Build history of the part. All positions in model axes, mm. A direction names the side the tool comes from. Give positions to 0.01 mm unless a question says otherwise; leave off trailing zeros. Write each loop counter-clockwise with the first axis right and the second up, starting at its lowest first coordinate (ties: lowest second). Pieces come first, ordered by that corner, then holes. Notation, with made-up numbers: (-5, 86.25) - (16, 86.25) arc R29 cw to (16, 113.25) - close; hole circle Ø9 at (-25.5, 9.5). An arc over 180 degrees is marked (long way). Use one line per item in the form item = value. Start each with the question number.
from build123d import *

# Parameters (mm, degrees)
SKETCH2_R           = 1.7
BOSS_EXTRUDE1_DEPTH = 1.625
SKETCH3_W           = 16
SKETCH3_H           = 12.05
BOSS_EXTRUDE2_DEPTH = 10.7
SKETCH4_W           = 14
SKETCH4_H           = 8.9
BOSS_EXTRUDE3_DEPTH = 6.25
SKETCH5_W           = 3.2
SKETCH5_H           = 8.9
BOSS_EXTRUDE4_DEPTH = 4.55
SKETCH6_R           = 3.95
BOSS_EXTRUDE5_DEPTH = 10.8
SKETCH7_R           = 2.43
SKETCH7_R_2         = 1.75
SKETCH7_W           = 4.5
SKETCH7_H           = 45
SKETCH7_W_2         = 20
SKETCH7_H_2         = 2.75
SKETCH7_W_3         = 24.5
SKETCH7_W_4         = 4.25
SKETCH7_H_3         = 7
BOSS_EXTRUDE6_DEPTH = 2.5
SKETCH8_W           = 25.8
SKETCH8_H           = 2.5
SKETCH8_W_2         = 20.65
SKETCH8_W_3         = 5
SKETCH8_H_2         = 46
SKETCH8_H_3         = 7.45
SKETCH8_W_4         = 7.45
SKETCH8_H_4         = 5
BOSS_EXTRUDE7_DEPTH = 8.25


with BuildPart() as part:
    # Sketch2 → Boss-Extrude1 (new body)
    with BuildSketch(Plane(origin=(0, 0, 0), x_dir=(1, 0, 0), z_dir=(0, 1, 0))):
        Polygon((99.1, 0), (99.1, 1.75), (101.35, 4), (101.35, 39), (99.1, 41.25), (99.1, 50.75), (96.45, 53.4), (0, 53.4), (0, 0), align=None)
        with Locations((96.65, 2.5)):
            Circle(SKETCH2_R, mode=Mode.SUBTRACT)
        with Locations((90.65, 50.95)):
            Circle(SKETCH2_R, mode=Mode.SUBTRACT)
        with Locations((15.45, 50.95)):
            Circle(SKETCH2_R, mode=Mode.SUBTRACT)
        with Locations((14.3, 2.5)):
            Circle(SKETCH2_R, mode=Mode.SUBTRACT)
        with Locations((66.2, 32.3)):
            Circle(SKETCH2_R, mode=Mode.SUBTRACT)
        with Locations((66.2, 7.7)):
            Circle(SKETCH2_R, mode=Mode.SUBTRACT)
    extrude(amount=BOSS_EXTRUDE1_DEPTH)

    # Sketch3 → Boss-Extrude2 (add)
    with BuildSketch(Plane(origin=(0, 1.625, 0), x_dir=(1, 0, 0), z_dir=(0, 1, 0))):
        with Locations((1.65, 38.375)):
            Rectangle(SKETCH3_W, SKETCH3_H)
    extrude(amount=BOSS_EXTRUDE2_DEPTH)

    # Sketch4 → Boss-Extrude3 (add)
    with BuildSketch(Plane(origin=(0, 1.625, 0), x_dir=(1, 0, 0), z_dir=(0, 1, 0))):
        with Locations((5.5, 8.45)):
            Rectangle(SKETCH4_W, SKETCH4_H)
    extrude(amount=BOSS_EXTRUDE3_DEPTH)

    # Sketch5 → Boss-Extrude4 (add)
    with BuildSketch(Plane(origin=(0, 7.875, 0), x_dir=(1, 0, 0), z_dir=(0, 1, 0))):
        with Locations((0.1, 8.45)):
            Rectangle(SKETCH5_W, SKETCH5_H)
    extrude(amount=BOSS_EXTRUDE4_DEPTH)

    # Sketch6 → Boss-Extrude5 (add)
    with BuildSketch(Plane(origin=(1.7, 0, 0), x_dir=(0, 0, -1), z_dir=(1, 0, 0))):
        with Locations((8.45, 7.875)):
            Circle(SKETCH6_R)
    extrude(amount=BOSS_EXTRUDE5_DEPTH)

    # Sketch7 → Boss-Extrude6 (add)
    with BuildSketch(Plane.XZ):
        with Locations((9, -3.25)):
            Circle(SKETCH7_R)
        with Locations((6, -8)):
            Circle(SKETCH7_R)
        with Locations((12, -8)):
            Circle(SKETCH7_R)
        with Locations((4, -32.65)):
            Circle(SKETCH7_R_2)
        with Locations((4, -44.65)):
            Circle(SKETCH7_R_2)
        with Locations((95.35, -29.65)):
            Rectangle(SKETCH7_W, SKETCH7_H)
        with Locations((77.6, -51.025)):
            Rectangle(SKETCH7_W_2, SKETCH7_H_2)
        with Locations((54.6, -51.025)):
            Rectangle(SKETCH7_W_2, SKETCH7_H_2)
        with Locations((30.35, -51.025)):
            Rectangle(SKETCH7_W_3, SKETCH7_H_2)
        with Locations((82.35, -2.875)):
            Rectangle(SKETCH7_W_2, SKETCH7_H_2)
        with Locations((59.35, -2.875)):
            Rectangle(SKETCH7_W_2, SKETCH7_H_2)
        with Locations((36.35, -2.875)):
            Rectangle(SKETCH7_W_2, SKETCH7_H_2)
        with Locations((64.075, -24.8)):
            Rectangle(SKETCH7_W_4, SKETCH7_H_3)
    extrude(amount=BOSS_EXTRUDE6_DEPTH)

    # Sketch8 → Boss-Extrude7 (add)
    with BuildSketch(Plane(origin=(0, 1.625, 0), x_dir=(1, 0, 0), z_dir=(0, 1, 0))):
        with Locations((30.4, 51.15)):
            Rectangle(SKETCH8_W, SKETCH8_H)
        with Locations((54.525, 51.15)):
            Rectangle(SKETCH8_W_2, SKETCH8_H)
        with Locations((77.275, 51.15)):
            Rectangle(SKETCH8_W_2, SKETCH8_H)
        with Locations((95.35, 29.4)):
            Rectangle(SKETCH8_W_3, SKETCH8_H_2)
        with Locations((36.825, 2.5)):
            Rectangle(SKETCH8_W_2, SKETCH8_H)
        with Locations((59.675, 2.5)):
            Rectangle(SKETCH8_W_2, SKETCH8_H)
        with Locations((82.525, 2.5)):
            Rectangle(SKETCH8_W_2, SKETCH8_H)
        with Locations((65.45, 24.325)):
            Rectangle(SKETCH8_W_3, SKETCH8_H_3)
        with Locations((18.225, 46.4)):
            Rectangle(SKETCH8_W_4, SKETCH8_H_4)
    extrude(amount=BOSS_EXTRUDE7_DEPTH)


solid = part.part
(1) Pin check, flat tips, straight feed: pin 1 Ø2 at (x, y) = (29, -1.5) entering from +Z; pin 2 Ø0.8 at (x, y) = (95, -2) entering from -Z; pin 3 Ø6.5 at (x, y) = (30.5, 6.5) entering from +Z. Stop position of each tip, or through.
(2) Which spindle directions (+Z, -Z, +X, -X, +Y, -Y) get a long thin tool onto all of the face, cutting with end or side? Do faces 1 (the flat face through (54, 6, -52.4)), 2 (the flat face through (4, 6, -12.9)), 3 (the flat face through (44.2, 6, -51)), 4 (the flat face through (18, 6, -43.9)), 5 (the flat face through (92.85, 6, -2)). Say none if no direction does.
(3) Two-plate mould, pull along X, no slides. Class faces 6 (the flat face through (92.85, 6, -29)), 7 (the flat face through (97.6, -1, -30)), 8 (the flat face through (59, -2.5, -3)): +X half, -X half, draft (parallel to the pull), parting line (faces both ways), or undercut.
(4) Wall check: line 1 (Z direction, x = 66.2, y = 0.5); line 2 (Z direction, x = 68, y = -0.5); line 3 (Z direction, x = 90.65, y = 1.2). Give the ranges that are in metal, low to high. Write a range as from..to.
(5) Cut at A-A, the plane x = 74.5. Give the cut face in (y, z) (3 decimals).
Solution:
q1.pin_1 = -1.5
q1.pin_2 = -52.15
q1.pin_3 = -1.25
q2.face_1 = -Z, +X, -X, +Y
q2.face_2 = -X, +Y
q2.face_3 = -Z, +Y
q2.face_4 = +Z, +Y
q2.face_5 = +Z, +X, +Y
q3.face_6 = undercut
q3.face_7 = +X half
q3.face_8 = draft
q4.line_1 = -53.4..-34, -30.6..-9.4, -6..0
q4.line_2 = -52.4..-49.65, -4.25..-1.5
q4.line_3 = -53.4..-52.65, -49.25..0
q5.outline = (-2.5, -52.4) - (0, -52.4) - (0, -53.4) - (1.625, -53.4) - (1.625, -52.4) - (9.875, -52.4) - (9.875, -49.9) - (1.625, -49.9) - (1.625, -3.75) - (9.875, -3.75) - (9.875, -1.25) - (1.625, -1.25) - (1.625, 0) - (0, 0) - (0, -1.5) - (-2.5, -1.5) - (-2.5, -4.25) - (0, -4.25) - (0, -49.65) - (-2.5, -49.65) - close
